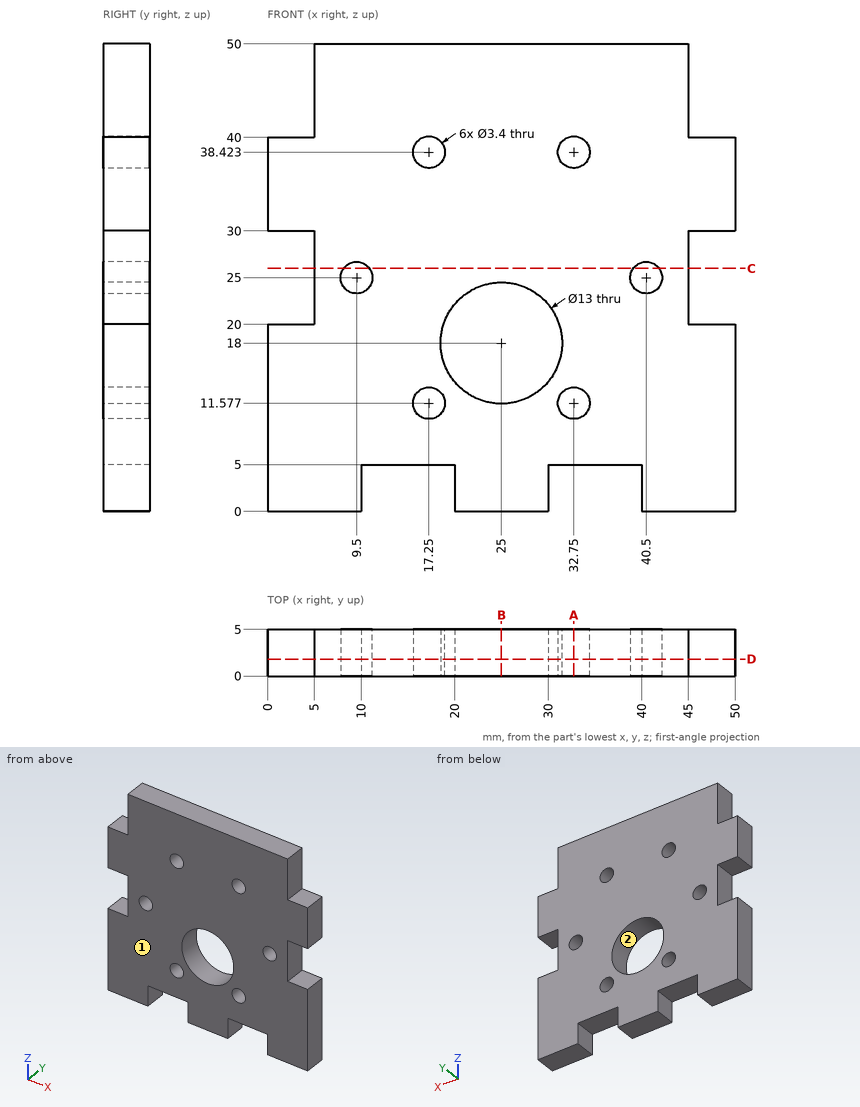
Print and shaded views of the part. All mm, measured from the part's lowest x, y and z. Give positions to 0.01 mm unless a question says otherwise; leave off trailing zeros. Order: outer loops, then holes, each group sorted by start corner. A loop starts at its lowest first (then second) coordinate and runs counter-clockwise, first axis right, second up. Notation, with made-up numbers: M 0,9.25 L 27,9.25 A18 cw 27,24.25 Z; hole C 25,-23 d7. An arc over 180 degrees is marked long. Use one line per item in the form item = value.
Q1. Slice it at A-A, the plane x = 32.75. Write the cut outline in (y, z).
Conclusion:
outline = M 0,5 L 5,5 L 5,9.88 L 0,9.88 Z; M 0,13.28 L 5,13.28 L 5,36.72 L 0,36.72 Z; M 0,40.12 L 5,40.12 L 5,50 L 0,50 Z
Q2. Slice it at D-D, the plane y = 1.8. State how many separate pieces and enclosed holes the cut face has, and give its area (3 significant figures).
Conclusion:
separate_pieces = 1
enclosed_holes = 7
area = 2,010 mm2
Q3. Pin check, flat tips, straight feed: P1, Ø1.5, axis at x = 3, y = 1.5, coming from the +Z side; P2, Ø1.5, axis at x = 33, y = 1.5, coming from the -Z side. Stop position of each tip, or through.
Conclusion:
P1 = 40
P2 = 5
Q4. Wall check: probe 1 along X at (y, z) = (2.35, 25); probe 2 along X at (y, z) = (1.75, 3.5); probe 3 along Z at (x, y) = (17.25, 3.5). Give the ranges that are in metal, low to high.
Conclusion:
probe_1 = 5 to 7.8, 11.2 to 38.8, 42.2 to 45
probe_2 = 0 to 10, 20 to 30, 40 to 50
probe_3 = 5 to 9.88, 13.28 to 36.72, 40.12 to 50
Q5. Slice it at C-C, the plane z = 26. Write the cut outline in (x, y) (1 decimal).
Conclusion:
outline = M 5,0 L 8.1,0 L 8.1,5 L 5,5 Z; M 10.9,0 L 39.1,0 L 39.1,5 L 10.9,5 Z; M 41.9,0 L 45,0 L 45,5 L 41.9,5 Z
Q6. Pull direction X, two halves, no side cores. Call the marked faces 1 and 2: released by +X, released by -X, zero draft, split by the parting line, or undercut.
Conclusion:
face_1 = zero draft
face_2 = undercut
Q7. Slice it at B-B, the plane x = 25. Write the cut outline in (y, z).
Conclusion:
outline = M 0,0 L 5,0 L 5,11.5 L 0,11.5 Z; M 0,24.5 L 5,24.5 L 5,50 L 0,50 Z
